```python
from build123d import *

# Parameters (mm, degrees)
SKETCH1_R           = 69.85
BOSS_EXTRUDE1_DEPTH = 6.35
SKETCH2_R           = 69.85
BOSS_EXTRUDE2_DEPTH = 6.35
SKETCH4_R           = 6.35
CUT_EXTRUDE1_DEPTH  = 6.35
SKETCH5_R           = 26.19375
SKETCH5_R_2         = 12.7
CUT_EXTRUDE2_DEPTH  = 6.35
SKETCH6_R           = 36.83
SKETCH6_R_2         = 31.75
CUT_EXTRUDE3_DEPTH  = 6.35
CUT_EXTRUDE4_START  = 8.505524
SKETCH8_R           = 0.508
CUT_EXTRUDE4_DEPTH  = 15.251285
SKETCH9_R           = 0.508
CUT_EXTRUDE5_DEPTH  = 12.7
CUT_EXTRUDE6_START  = 11.006381
SKETCH11_R          = 0.508
CUT_EXTRUDE6_DEPTH  = 7.918937
CIRPATTERN1_COUNT   = 16
SKETCH12_R          = 2.54
CUT_EXTRUDE7_DEPTH  = 13.7
CIRPATTERN2_COUNT   = 18
SKETCH13_R          = 10.3632
SKETCH13_R_2        = 7.7216
CUT_EXTRUDE8_DEPTH  = 1.3208
SKETCH14_R          = 30.2133
SKETCH14_R_2        = 27.5717
CUT_EXTRUDE9_DEPTH  = 1.3208
SKETCH16_R          = 46.0883
SKETCH16_R_2        = 43.4467
CUT_EXTRUDE10_DEPTH = 1.3208
SKETCH20_R          = 69.85
CUT_EXTRUDE11_DEPTH = 6.35


with BuildPart() as part:
    # Sketch1 → Boss-Extrude1 (new body)
    with BuildSketch(Plane(origin=(0, 0, 0), x_dir=(1, 0, 0), z_dir=(0, 1, 0))):
        Circle(SKETCH1_R)
    extrude(amount=BOSS_EXTRUDE1_DEPTH)

    # Sketch2 → Boss-Extrude2 (add)
    with BuildSketch(Plane.XZ):
        Circle(SKETCH2_R)
    extrude(amount=BOSS_EXTRUDE2_DEPTH)

    # Sketch4 → Cut-Extrude1 (cut)
    with BuildSketch(Plane(origin=(0, 6.35, 0), x_dir=(1, 0, 0), z_dir=(0, 1, 0))):
        Circle(SKETCH4_R)
    extrude(amount=-CUT_EXTRUDE1_DEPTH, mode=Mode.SUBTRACT)

    # Sketch5 → Cut-Extrude2 (cut)
    with BuildSketch(Plane(origin=(0, 6.35, 0), x_dir=(1, 0, 0), z_dir=(0, 1, 0))):
        Circle(SKETCH5_R)
        Circle(SKETCH5_R_2, mode=Mode.SUBTRACT)
    extrude(amount=-CUT_EXTRUDE2_DEPTH, mode=Mode.SUBTRACT)

    # Sketch6 → Cut-Extrude3 (cut)
    with BuildSketch(Plane(origin=(0, 6.35, 0), x_dir=(1, 0, 0), z_dir=(0, 1, 0))):
        Circle(SKETCH6_R)
        Circle(SKETCH6_R_2, mode=Mode.SUBTRACT)
    extrude(amount=-CUT_EXTRUDE3_DEPTH, mode=Mode.SUBTRACT)

    # Sketch8 → Cut-Extrude4 (cut)
    with BuildSketch(Plane(origin=(-1.740960292, 3.015431679, 0), x_dir=(-0.866025404, -0.5, 0), z_dir=(-0.5, 0.866025404, 0)).offset(CUT_EXTRUDE4_START)):
        with Locations((33.970863359, 0)):
            Circle(SKETCH8_R)
    cut_extrude4 = extrude(amount=CUT_EXTRUDE4_DEPTH, mode=Mode.SUBTRACT)

    # Sketch9 → Cut-Extrude5 (cut)
    with BuildSketch(Plane.XZ.offset(6.35)):
        with Locations((-26.67, 0)):
            Circle(SKETCH9_R)
        with Locations((-17.78, 0)):
            Circle(SKETCH9_R)
    cut_extrude5 = extrude(amount=-CUT_EXTRUDE5_DEPTH, mode=Mode.SUBTRACT)

    # Sketch11 → Cut-Extrude6 (cut)
    with BuildSketch(Plane(origin=(-10.621968306, -18.397788783, 0), x_dir=(0.866025404, -0.5, 0), z_dir=(0.5, 0.866025404, 0)).offset(CUT_EXTRUDE6_START)):
        with Locations((-4.52396584, 0)):
            Circle(SKETCH11_R)
    cut_extrude6 = extrude(amount=CUT_EXTRUDE6_DEPTH, mode=Mode.SUBTRACT)

    # CirPattern1: Cut-Extrude4, Cut-Extrude5, Cut-Extrude6 ×16 about axis
    cirpattern1_axis = Axis((0, 0, 0), (0, 1, 0))
    for i in range(1, CIRPATTERN1_COUNT):
        add(cut_extrude4.rotate(cirpattern1_axis, i * 360 / CIRPATTERN1_COUNT), mode=Mode.SUBTRACT)
        add(cut_extrude5.rotate(cirpattern1_axis, i * 360 / CIRPATTERN1_COUNT), mode=Mode.SUBTRACT)
        add(cut_extrude6.rotate(cirpattern1_axis, i * 360 / CIRPATTERN1_COUNT), mode=Mode.SUBTRACT)

    # Sketch12 → Cut-Extrude7 (cut, through all)
    with BuildSketch(Plane(origin=(0, 6.35, 0), x_dir=(1, 0, 0), z_dir=(0, 1, 0))):
        with Locations((63.5, 0)):
            Circle(SKETCH12_R)
    cut_extrude7 = extrude(amount=-CUT_EXTRUDE7_DEPTH, mode=Mode.SUBTRACT)

    # CirPattern2: Cut-Extrude7 ×18 about axis
    cirpattern2_axis = Axis((0, 0, 0), (0, 1, 0))
    for i in range(1, CIRPATTERN2_COUNT):
        add(cut_extrude7.rotate(cirpattern2_axis, i * 360 / CIRPATTERN2_COUNT), mode=Mode.SUBTRACT)

    # Sketch13 → Cut-Extrude8 (cut)
    with BuildSketch(Plane(origin=(0, 6.35, 0), x_dir=(1, 0, 0), z_dir=(0, 1, 0))):
        Circle(SKETCH13_R)
        Circle(SKETCH13_R_2, mode=Mode.SUBTRACT)
    extrude(amount=-CUT_EXTRUDE8_DEPTH, mode=Mode.SUBTRACT)

    # Sketch14 → Cut-Extrude9 (cut)
    with BuildSketch(Plane(origin=(0, 6.35, 0), x_dir=(1, 0, 0), z_dir=(0, 1, 0))):
        Circle(SKETCH14_R)
        Circle(SKETCH14_R_2, mode=Mode.SUBTRACT)
    extrude(amount=-CUT_EXTRUDE9_DEPTH, mode=Mode.SUBTRACT)

    # Sketch16 → Cut-Extrude10 (cut)
    with BuildSketch(Plane(origin=(0, 6.35, 0), x_dir=(1, 0, 0), z_dir=(0, 1, 0))):
        Circle(SKETCH16_R)
        Circle(SKETCH16_R_2, mode=Mode.SUBTRACT)
    extrude(amount=-CUT_EXTRUDE10_DEPTH, mode=Mode.SUBTRACT)

    # Sketch20 → Cut-Extrude11 (cut)
    with BuildSketch(Plane(origin=(0, 6.35, 0), x_dir=(1, 0, 0), z_dir=(0, 1, 0))):
        Circle(SKETCH20_R)
    extrude(amount=-CUT_EXTRUDE11_DEPTH, mode=Mode.SUBTRACT)


solid = part.part
```
Could you check a few things on this model? Use its own coordinates, in mm. Round coordinates to 2 decimals unless told otherwise and drop trailing zeros. Write each loop counter-clockwise with the first axis right and the second up, starting at its lowest first coordinate (ties: lowest second). Pieces come first, ordered by that corner, then holes.
(1) Suppose I cut it at C-C on z = 49. Write out the boundary of the cut face in (x, y).
Findings below:
outline: (-49.78, -6.35) - (49.78, -6.35) - (49.78, 0) - (-49.78, 0) - close
(2) Thinking about a two-plate mould opening in X: for faces 1 (the face through (-1, 0, -1)), 2 (the face through (26.13, -2.97, 26.09)), which applies, +X half, -X half, draft (parallel to the pull), parting line (faces both ways), or undercut?
Findings below:
face 1: draft
face 2: undercut
(3) For pin 1 (0.9 mm diameter, centred on x = 18.86, z = -18.86, fed in from +Y); pin 2 (2 mm diameter, centred on x = -19.5, y = -1, fed in from -Z); pin 3 (1 mm diameter, centred on x = 9, y = -5, fed in from -Z); pin 4 (1 mm diameter, centred on x = -16.5, y = -3, fed in from -Z), each with a flat end and sliding along its axis, tell me the tip position at first contact or that it passes through.
Findings below:
pin 1: passes through
pin 2: stops at z = -67.36
pin 3: stops at z = -69.33
pin 4: stops at z = -67.99
(4) Suppose I cut it at B-B on x = -21. Write out the boundary of the cut face in (y, z).
Findings below:
outline: (-6.35, -66.62) - (0, -66.62) - (0, 66.62) - (-6.35, 66.62) - close
(5) If I drill on probe 1 along Z at (x, y) = (31.75, -2.75); probe 2 along X at (y, z) = (-0.75, -35.5); probe 3 along X at (y, z) = (-3.25, -20), over which ranges is the centre line in solid material (lowest first)?
Findings below:
probe 1: z = -62.22 to -57.53, -52.45 to 52.45, 57.53 to 62.22
probe 2: x = -60.16 to -15.23, -14.4 to 14.4, 15.23 to 60.16
probe 3: x = -66.93 to -61.54, -57.8 to 57.8, 61.54 to 66.93
(6) Suppose I cut it at A-A on y = -3.75. State how many separate pieces and enclosed holes the cut face has, and give its area (3 significant figures).
Findings below:
separate pieces: 1
enclosed holes: 82
area: 14,900 mm2
